Read the model definition and answer for the solid it produces. Units are mm, in the model's axes. Round coordinates to 2 decimals unless told otherwise and drop trailing zeros. Order: outer loops, then holes, each group sorted by start corner. A loop starts at its lowest first (then second) coordinate and runs counter-clockwise, first axis right, second up.
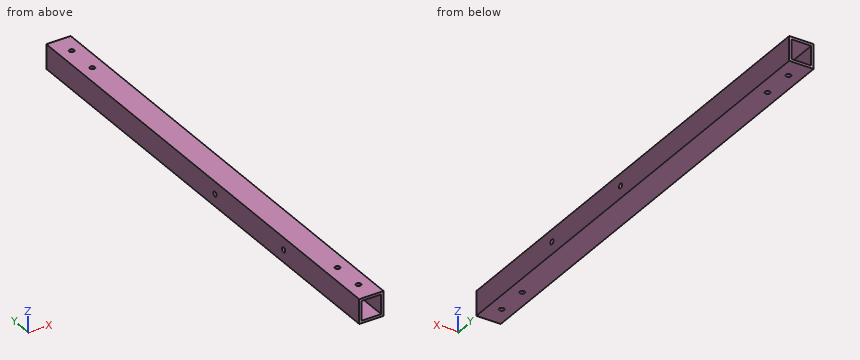
from build123d import *

# Parameters (mm, degrees)
SKETCH1_W              = 15
SKETCH1_H              = 15
SKETCH1_W_2            = 12
SKETCH1_H_2            = 12
EXTRUDE_THIN1_DEPTH    = 300
SKETCH2_R              = 1.5
CUT_EXTRUDE1_DEPTH     = 301.749064836
CUT_EXTRUDE2_OUTLINE_R = 1.5
CUT_EXTRUDE2_DEPTH     = 15


# Read off the part's stored shape, not the designer's step: Cut-Extrude2
with BuildPart() as part:
    # Sketch1 → Extrude-Thin1 (new body)
    with BuildSketch(Plane(origin=(0, 0, 0), x_dir=(1, 0, 0), z_dir=(0, 1, 0))):
        with Locations((7.5, 7.5)):
            Rectangle(SKETCH1_W, SKETCH1_H)
        with Locations((7.5, 7.5)):
            Rectangle(SKETCH1_W_2, SKETCH1_H_2, mode=Mode.SUBTRACT)
    extrude(amount=EXTRUDE_THIN1_DEPTH)

    # Sketch2 (on Front Plane) → Cut-Extrude1 (cut, through all)
    with BuildSketch(Plane.XY):
        with Locations((7.5, 12.5)):
            Circle(SKETCH2_R)
        with Locations((7.5, 32.5)):
            Circle(SKETCH2_R)
        with Locations((7.5, 267.5)):
            Circle(SKETCH2_R)
        with Locations((7.5, 287.5)):
            Circle(SKETCH2_R)
    extrude(amount=-CUT_EXTRUDE1_DEPTH, mode=Mode.SUBTRACT)

    # Cut-Extrude2 outline → Cut-Extrude2 (cut)
    with BuildSketch(Plane.YZ):
        with Locations((138.290000004, -7.5)):
            Circle(CUT_EXTRUDE2_OUTLINE_R)
        with Locations((72.500000004, -7.5)):
            Circle(CUT_EXTRUDE2_OUTLINE_R)
    extrude(amount=CUT_EXTRUDE2_DEPTH, mode=Mode.SUBTRACT)


solid = part.part
Q1. A flat-ended cylindrical pin translates along its axis: pin 1 (6 mm diameter, centred on x = 2, z = -6.5, fed in from -Y). Find the tip coordinate at first contact, or state that the pin passes through.
Outcome:
pin 1: stops at y = 0
Q2. Straight lines are drawn through the part: probe 1 along Y at (x, z) = (7.5, -13.85); probe 2 along Y at (x, z) = (14.55, -7.5); probe 3 along Z at (x, y) = (9.75, 87). For each, find the intervals that lie inside material, in ascending order.
Outcome:
probe 1: y = 0 to 11, 14 to 31, 34 to 266, 269 to 286, 289 to 300
probe 2: y = 0 to 71, 74 to 136.79, 139.79 to 300
probe 3: z = -15 to -13.5, -1.5 to 0
Q3. A cutting plane is placed at A-A, the plane y = 58. Give the vertices of the cut face in (x, z), plus the area to 3 significant figures.
Outcome:
outline: (0, -15) - (15, -15) - (15, 0) - (0, 0) - close; hole (1.5, -13.5) - (13.5, -13.5) - (13.5, -1.5) - (1.5, -1.5) - close
area: 81.0 mm2
